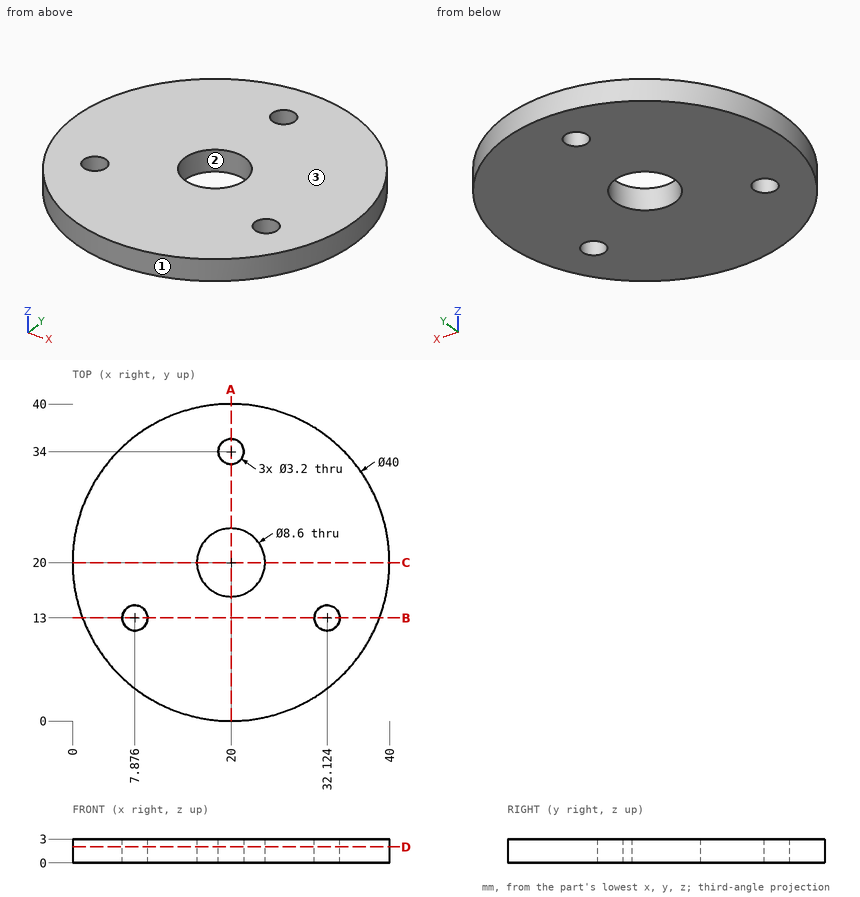
Job drawing, mm, ordinate dimensions from the low corner. One solid piece. Coordinates: 2 decimals unless noted, no trailing zeros. Loops run counter-clockwise (first coordinate to the right, second up) from the corner with the lowest first, then second, coordinate; pieces in that order, holes last. Notation, with made-up numbers: (-5, 33) - (27, 33) arc R22 cw to (27, 41) - close; hole circle Ø5 at (7.25, 70.5). An arc over 180 degrees is marked (long way). Answer as a JSON object with one key per item and string values. Group by question number.
(1) Cut at A-A (x = 20). Give the cut face in (y, z).
(2) Probe line 1 along Y through (x, z) = (20, 1.1); line 2 along X through (y, z) = (22.5, 1.8); line 3 along X through (y, z) = (3, 1.9) (1 decimal). List the from-to ranges inside material, lowest first.
(3) Cut at D-D (z = 2). Give the cut face in (x, y) (1 decimal), then the cut area to 3 significant figures.
(4) Cut at C-C (y = 20). Give the cut face in (x, z).
(5) Two-plate mould, pull along X, no slides. Class the marked faces 1, 2 and 3: released by +X, released by -X, zero draft, split by the parting line, or undercut.
(6) Flat gauge pins, fed straight in: pin 1 (3 mm diameter, centred on x = 7.88, y = 13, fed in from -Z); pin 2 (1 mm diameter, centred on y = 31, z = 1, fed in from +X). Where does each tip first touch, or does it go through?
(7) Cut at B-B (y = 13). Give the cut face in (x, z) (1 decimal).
Geometry says:
{
 "1": {"outline": "(0, 0) - (15.7, 0) - (15.7, 3) - (0, 3) - close; (24.3, 0) - (32.4, 0) - (32.4, 3) - (24.3, 3) - close; (35.6, 0) - (40, 0) - (40, 3) - (35.6, 3) - close"},
 "2": {"line 1": "y = 0 to 15.7, 24.3 to 32.4, 35.6 to 40", "line 2": "x = 0.16 to 16.5, 23.5 to 39.84", "line 3": "x = 9.5 to 30.5"},
 "3": {"outline": "circle Ø40 at (20, 20); hole circle Ø3.2 at (7.9, 13); hole circle Ø8.6 at (20, 20); hole circle Ø3.2 at (20, 34); hole circle Ø3.2 at (32.1, 13)", "area": "1,170 mm^2"},
 "4": {"outline": "(0, 0) - (15.7, 0) - (15.7, 3) - (0, 3) - close; (24.3, 0) - (40, 0) - (40, 3) - (24.3, 3) - close"},
 "5": {"face 1": "split by the parting line", "face 2": "undercut", "face 3": "zero draft"},
 "6": {"pin 1": "passes through", "pin 2": "stops at x = 37.02"},
 "7": {"outline": "(1.3, 0) - (6.3, 0) - (6.3, 3) - (1.3, 3) - close; (9.5, 0) - (30.5, 0) - (30.5, 3) - (9.5, 3) - close; (33.7, 0) - (38.7, 0) - (38.7, 3) - (33.7, 3) - close"}
}
